```python
from build123d import *

# Parameters (mm, degrees)
F0_W     = 7.9375
F0_H     = 8.1661
F0_R     = 1.5875
F1_DEPTH = 14.2875
F2_R     = 2.54
F3_R     = 1.19126
F4_DEPTH = 2.54
F3_R_2   = 0.6604
F5_DEPTH = 3.81


with BuildPart() as f1:
    # F0 (on Front) → F1 (new body)
    with BuildSketch(Plane.XZ):
        with Locations((3.96875, 4.08305)):
            Rectangle(F0_W, F0_H)
        with Locations((3.97002, 4.7625)):
            Circle(F0_R, mode=Mode.SUBTRACT)
    extrude(amount=-F1_DEPTH)

    # F2
    f2_edges = [f1.edges().sort_by_distance(p)[0] for p in [
        (0, 7.14375, 8.1661),
        (7.9375, 7.14375, 8.1661),
    ]]
    fillet(f2_edges, radius=F2_R)

    # F3 (on Top) → F4 (cut)
    with BuildSketch(Plane.XY):
        with Locations((3.97002, 8.73252)):
            Circle(F3_R)
    extrude(amount=F4_DEPTH, mode=Mode.SUBTRACT)

    # F3 (on Top) → F5 (cut)
    with BuildSketch(Plane.XY):
        with Locations((3.97002, 2.38252)):
            Circle(F3_R_2)
    extrude(amount=F5_DEPTH, mode=Mode.SUBTRACT)


solid = f1.part
```
For this review, take the finished solid that the model builds, in its own axes (mm). A direction names the side the tool comes from. Coordinates: 2 decimals unless noted, no trailing zeros. Order: outer loops, then holes, each group sorted by start corner. A loop starts at its lowest first (then second) coordinate and runs counter-clockwise, first axis right, second up. Notation, with made-up numbers: (-38.75, -19.75) - (-14.75, -19.75) arc R22 cw to (-14.75, 13.25) - close; hole circle Ø1 at (-13, 45.25). An arc over 180 degrees is marked (long way). Answer as a JSON object with one key per item and string values. Group by question number.
1. We need section D-D on z = 1.75. State the section outline as (x, y) points.
2. The part is to be moulded in two halves that separate along X. For faces 1 (the cylindrical face through (4.52, 7.676, 1.252)), 2 (the flat face through (0, 7, 3)), 3 (the flat face through (7.938, 7, 3)), say which applies: pulls with the +X half, pulls with the -X half, needs draft (parallel to the pull), parting line crosses it, or undercut.
3. We need section B-B on z = 5. State the section outline as (x, y) points, then the cut area to 3 significant figures.
4. We need section A-A on x = 4.25. State the section outline as (y, z) points, then the cut area to 3 significant figures.
5. We need section C-C on y = 9.25. State the section outline as (x, z) points (1 decimal).
6. For faces 4 (the cylindrical face through (0.72, 7.24, 7.4)), 5 (the cylindrical face through (3.31, 2.41, 1.64)), list the 3-axis set-ups (+Z, -Z, +X, -X, +Y, -Y) from which the entire face can be reached by the end or side of a thin tool; tool diameter is ignored.
7. For probe 1 along Y at (x, z) = (3.5, 0.5); probe 2 along X at (y, z) = (7.5, 6); probe 3 along Z at (x, y) = (4.5, 11.5), list the stretches that pass through material, from the lowest coordinate up.
8. Clearance check with a flat-ended pin moving along its axis: P1, Ø2.5, axis at x = 3.97, z = 4.76, coming from the -Y side. State where the tip first meets the part, or that it passes through.
Final values:
{
 "1": {"outline": "(0, 0) - (7.94, 0) - (7.94, 14.29) - (0, 14.29) - close; hole circle Ø2.38 at (3.97, 8.73); hole circle Ø1.32 at (3.97, 2.38)"},
 "2": {"face 1": "undercut", "face 2": "pulls with the -X half", "face 3": "pulls with the +X half"},
 "3": {"outline": "(0, 0) - (2.4, 0) - (2.4, 14.29) - (0, 14.29) - close; (5.54, 0) - (7.94, 0) - (7.94, 14.29) - (5.54, 14.29) - close", "area": "68.6 mm²"},
 "4": {"outline": "(0, 0) - (1.78, 0) - (1.78, 3.2) - (0, 3.2) - close; (0, 6.33) - (14.29, 6.33) - (14.29, 8.17) - (0, 8.17) - close; (2.98, 0) - (7.57, 0) - (7.57, 2.54) - (9.89, 2.54) - (9.89, 0) - (14.29, 0) - (14.29, 3.2) - (2.98, 3.2) - close", "area": "62.3 mm²"},
 "5": {"outline": "(0, 0) - (2.9, 0) - (2.9, 2.5) - (5, 2.5) - (5, 0) - (7.9, 0) - (7.9, 5.6) arc R2.5 ccw to (5.4, 8.2) - (2.5, 8.2) arc R2.5 ccw to (0, 5.6) - close; hole circle Ø3.2 at (4, 4.8)"},
 "6": {"face 4": "+Z, -X, +Y, -Y", "face 5": "-Z"},
 "7": {"probe 1": "0 to 1.92, 2.85 to 7.64, 9.83 to 14.29", "probe 2": "0.03 to 2.98, 4.96 to 7.91", "probe 3": "0 to 3.27, 6.26 to 8.17"},
 "8": {"P1": "through"}
}
